```python
from build123d import *

# Parameters (mm, degrees)
SKETCH004_W             = 12
SKETCH004_H             = 10
SKETCH004_R             = 1.05
PAD004_DEPTH            = 5.4
PAD005_START            = 1
PAD005_DEPTH            = 3.4
SKETCH006_R             = 1
PAD006_DEPTH            = 12
PAD007_START            = 1
PAD007_DEPTH            = 3.4
BODY003_PLACEMENT_ANGLE = 324


with BuildPart() as part:
    # Sketch004 → Pad004 (new body)
    with BuildSketch(Plane.XY):
        with Locations((6, 5)):
            Rectangle(SKETCH004_W, SKETCH004_H)
        with Locations((2.05, 2.171592)):
            Circle(SKETCH004_R, mode=Mode.SUBTRACT)
        with Locations((8.95, 7.95)):
            Circle(SKETCH004_R, mode=Mode.SUBTRACT)
    extrude(amount=PAD004_DEPTH)

    # Sketch005 → Pad005 (join)
    with BuildSketch(Plane.XY.offset(PAD005_START)):
        with BuildLine():
            Line((-4.242641, 12.828427), (0.353553, 8.232233))
            Line((0.353553, 8.232233), (1.767767, 9.646447))
            Line((1.767767, 9.646447), (-2.828427, 14.242641))
            ThreePointArc((-2.828427, 14.242641), (-4.242641, 14.242641), (-4.242641, 12.828427))
        make_face()
    extrude(amount=PAD005_DEPTH)

    # Sketch006 (on Face1 of Pad005) → Pad006 (join)
    with BuildSketch(Plane.XZ):
        with Locations((3.5, 2.7)):
            Circle(SKETCH006_R)
        with Locations((6, 2.7)):
            Circle(SKETCH006_R)
        with Locations((8.5, 2.7)):
            Circle(SKETCH006_R)
    extrude(amount=PAD006_DEPTH)

    # Sketch007 → Pad007 (join)
    with BuildSketch(Plane.XY.offset(PAD007_START)):
        with BuildLine():
            Line((1.06066, 7.93934), (-5.43934, 7.93934))
            ThreePointArc((-5.43934, 9.93934), (-6.43934, 8.93934), (-5.43934, 7.93934))
            Line((-5.43934, 9.93934), (1.06066, 9.93934))
            Line((1.06066, 7.93934), (1.06066, 9.93934))
        make_face()
    extrude(amount=PAD007_DEPTH)


with BuildPart() as part_1:
    # Body003 placement: moved
    add(part.part.moved(Location((10.236799, 8.319416, 0))).rotate(Axis((10.236799, 8.319416, 0), (0, 0, -1)), BODY003_PLACEMENT_ANGLE))


solid = part_1.part
```
Work out the finished part from the listing and answer in its coordinate system (mm). A direction names the side the tool comes from. Round coordinates to 2 decimals unless told otherwise and drop trailing zeros. Write each loop counter-clockwise with the first axis right and the second up, starting at its lowest first coordinate (ties: lowest second). Pieces come first, ordered by that corner, then holes. Notation, with made-up numbers: (8.25, 87.25) - (57.25, 87.25) arc R15 ccw to (57.25, 112.25) - close; hole circle Ø10 at (32.5, 29). An arc over 180 degrees is marked (long way). Return JSON: item names as keys, results as strings. Group by question number.
Q1. The part is cut by section B-B on x = 2. Write down the section's boundary in (y, z), then the cut area to 3 significant figures.
Q2. Each of these flat-tipped pins is pushed along its axis until it touches: pin 1 Ø12 at (x, y) = (3.5, 7) entering from +Z; pin 2 Ø3 at (y, z) = (8.5, 1) entering from -X; pin 3 Ø5.5 at (x, y) = (1, 15) entering from -Z; pin 4 Ø1.9 at (x, y) = (12.8, 20.01) entering from -Z. Where does it stop, or does it pass through?
Q3. The mould has two halves that part along Y. Classify faces 1 (the flat face through (7.339, 12.308, 2.662)), 2 (the cylindrical face through (21.362, 9.09, 3)), 3 (the cylindrical face through (-1.564, 17.37, 2.676)): released by +Y, released by -Y, zero draft, split by the parting line, or undercut.
Q4. Find the intervals of material crossed by L1, parallel to X at y = 12.5, z = 2.95; L2, parallel to X at y = 20.25, z = 4.75; L3, parallel to X at y = 20, z = 4.5, in increasing order.
Q5. For faces 4 (the flat face through (3.401, 13.166, 2.676)), 5 (the flat face through (2.6, 17.7, 2.7)), 6 (the flat face through (1.25, 15.89, 2.68)), 7 (the flat face through (15.023, 11.797, 1.462)), determine the directions among +Z, -Z, +X, -X, +Y, -Y from which every point of the face is accessible in a straight line to the end or side of a thin tool.
Q6. The part is cut by section A-A on z = 2.1. Count the separate pieces of the cut face and the enclosed holes in it, then the cut area to 3 significant figures.
Q7. The part is cut by section C-C on x = 9. Write down the section's boundary in (y, z).
Solved:
{
 "1": {"outline": "(12.15, 1) - (14.62, 1) - (14.62, 4.4) - (12.15, 4.4) - close; (15.77, 1) - (17.8, 1) - (17.8, 4.4) - (15.77, 4.4) - close", "area": "15.3 mm²"},
 "2": {"pin 1": "z = 4.4", "pin 2": "x = 9.02", "pin 3": "z = 1", "pin 4": "through"},
 "3": {"face 1": "released by -Y", "face 2": "undercut", "face 3": "split by the parting line"},
 "4": {"L1": "-0.41 to 2.48, 7.2 to 15.99, 16.51 to 18.9", "L2": "9.64 to 11.78, 13.83 to 16.4", "L3": "9.3 to 11.75, 13.85 to 16.58"},
 "5": {"face 4": "+Z, -Z, -Y", "face 5": "+Z, -Z, +Y", "face 6": "+Z, -Z, -X", "face 7": "none"},
 "6": {"separate pieces": "1", "enclosed holes": "2", "area": "195 mm²"},
 "7": {"outline": "(10.02, 0) - (19.78, 0) - (19.78, 5.4) - (10.02, 5.4) - close"}
}
